```python
from build123d import *

# Parameters (mm, degrees)
BOSS_EXTRUDE1_DEPTH = 1.5
BOSS_EXTRUDE2_START = -10
BOSS_EXTRUDE2_DEPTH = 5
BOSS_EXTRUDE3_START = -50
BOSS_EXTRUDE3_DEPTH = 5
FILLET1_R           = 5
SKETCH4_R           = 1.1
CUT_EXTRUDE1_DEPTH  = 1.5
SKETCH5_R           = 0.85
CUT_EXTRUDE2_DEPTH  = 6


with BuildPart() as part:
    # Sketch1 → Boss-Extrude1 (new body)
    with BuildSketch(Plane(origin=(0, 0, 0), x_dir=(1, 0, 0), z_dir=(0, 1, 0))):
        with BuildLine():
            Line((2.414213562, 0), (69.385786438, 0))
            ThreePointArc((69.385786438, 0), (69.794034728, 0.211324865), (69.857190958, 0.666666667))
            ThreePointArc((69.857190958, 0.666666667), (70.092893219, 1.707106781), (71.133333333, 1.942809042))
            ThreePointArc((71.133333333, 1.942809042), (71.588675135, 2.005965272), (71.8, 2.414213562))
            Line((71.8, 2.414213562), (71.8, 34.385786438))
            ThreePointArc((71.8, 34.385786438), (71.588675135, 34.794034728), (71.133333333, 34.857190958))
            ThreePointArc((71.133333333, 34.857190958), (70.092893219, 35.092893219), (69.857190958, 36.133333333))
            ThreePointArc((69.857190958, 36.133333333), (69.794034728, 36.588675135), (69.385786438, 36.8))
            Line((69.385786438, 36.8), (2.414213562, 36.8))
            ThreePointArc((2.414213562, 36.8), (2.005965272, 36.588675135), (1.942809042, 36.133333333))
            ThreePointArc((1.942809042, 36.133333333), (1.707106781, 35.092893219), (0.666666667, 34.857190958))
            ThreePointArc((0.666666667, 34.857190958), (0.211324865, 34.794034728), (0, 34.385786438))
            Line((0, 34.385786438), (0, 2.414213562))
            ThreePointArc((0, 2.414213562), (0.211324865, 2.005965272), (0.666666667, 1.942809042))
            ThreePointArc((0.666666667, 1.942809042), (1.707106781, 1.707106781), (1.942809042, 0.666666667))
            ThreePointArc((1.942809042, 0.666666667), (2.005965272, 0.211324865), (2.414213562, 0))
        make_face()
    extrude(amount=BOSS_EXTRUDE1_DEPTH)

    # Sketch3 → Boss-Extrude2 (add)
    with BuildSketch(Plane.ZY.offset(BOSS_EXTRUDE2_START)):
        with BuildLine():
            Line((-12.854731747, 0), (-18.4, 0))
            ThreePointArc((-18.4, 0), (-13.582214371, -17.687731165), (-26.704575482, -4.886538603))
            Line((-26.704575482, -4.886538603), (-31.425470843, -1.179783346))
            Line((-31.425470843, -1.179783346), (-32.35181379, -2.359566693))
            Line((-32.35181379, -2.359566693), (-28.576454789, -5.323905182))
            ThreePointArc((-28.576454789, -5.323905182), (-14.871832802, -19.918830847), (-12.854731747, 0))
        make_face()
        with BuildLine():
            Line((-18.4, 0), (-30.499127896, 0))
            Line((-30.499127896, 0), (-25.871961194, -3.633161336))
            ThreePointArc((-25.871961194, -3.633161336), (-22.554216695, -0.956436127), (-18.4, 0))
        make_face()
    extrude(amount=-BOSS_EXTRUDE2_DEPTH)

    # Sketch3_3 → Boss-Extrude3 (add)
    with BuildSketch(Plane.ZY.offset(BOSS_EXTRUDE3_START)):
        with BuildLine():
            Line((-18.4, 0), (-30.499127896, 0))
            Line((-30.499127896, 0), (-25.871961194, -3.633161336))
            ThreePointArc((-25.871961194, -3.633161336), (-22.554216695, -0.956436127), (-18.4, 0))
        make_face()
        with BuildLine():
            Line((-12.854731747, 0), (-18.4, 0))
            ThreePointArc((-18.4, 0), (-13.582214371, -17.687731165), (-26.704575482, -4.886538603))
            Line((-26.704575482, -4.886538603), (-31.425470843, -1.179783346))
            Line((-31.425470843, -1.179783346), (-32.35181379, -2.359566693))
            Line((-32.35181379, -2.359566693), (-28.576454789, -5.323905182))
            ThreePointArc((-28.576454789, -5.323905182), (-14.871832802, -19.918830847), (-12.854731747, 0))
        make_face()
    extrude(amount=-BOSS_EXTRUDE3_DEPTH)

    # Fillet1
    fillet1_edges = [part.edges().sort_by_distance(p)[0] for p in [
        (12.5, 0, -12.854731747),
        (52.5, 0, -12.854731747),
    ]]
    fillet(fillet1_edges, radius=FILLET1_R)

    # Sketch4 → Cut-Extrude1 (cut)
    with BuildSketch(Plane(origin=(0, -17.173792622, -13.484528084), x_dir=(1, 0, 0), z_dir=(0, -0.7865222309713126, -0.6175619646544867))):
        with Locations(Location((12.5, -21.609183849, 0), (0, 0, 270))):
            Circle(SKETCH4_R)
        with Locations(Location((52.5, -21.609183849, 0), (0, 0, 270))):
            Circle(SKETCH4_R)
    extrude(amount=-CUT_EXTRUDE1_DEPTH, mode=Mode.SUBTRACT)

    # Sketch5 → Cut-Extrude2 (cut)
    with BuildSketch(Plane(origin=(0, -17.173792622, -13.484528084), x_dir=(1, 0, 0), z_dir=(0, -0.7865222309713126, -0.6175619646544867))):
        with Locations(Location((12.5, -21.609183849, 0), (0, 0, 270))):
            Circle(SKETCH5_R)
        with Locations(Location((52.5, -21.609183849, 0), (0, 0, 270))):
            Circle(SKETCH5_R)
    extrude(amount=-CUT_EXTRUDE2_DEPTH, mode=Mode.SUBTRACT)


solid = part.part
```
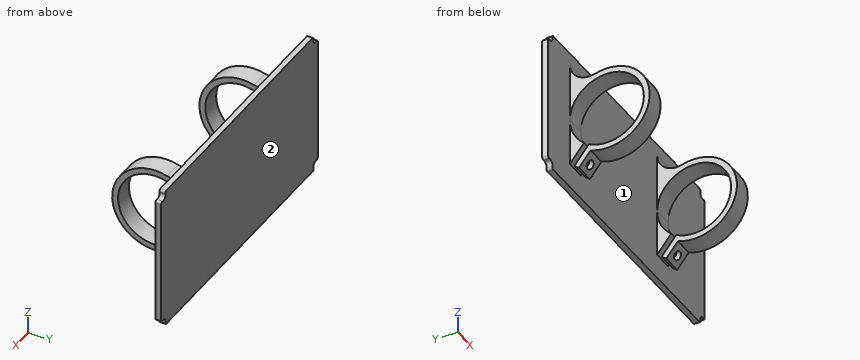
Part model, mm, in its own coordinate system. Face numbers are marked on the shaded views. Give positions to 0.01 mm unless a question says otherwise; leave off trailing zeros. Order: outer loops, then holes, each group sorted by start corner. A loop starts at its lowest first (then second) coordinate and runs counter-clockwise, first axis right, second up. Notation, with made-up numbers: M 27.25,48.25 L 65.25,48.25 A22 ccw 65.25,82.25 Z; hole C 64,73.5 d6. An arc over 180 degrees is marked long. Use a Markdown table: item, result. Add a question column.
(1) Probe line 1 along Y through (x, z) = (53.8, -18.4); line 2 along Z through (x, y) = (51.2, -9.5); line 3 along X through (y, z) = (-13.75, -9). List the from-to ranges inside material, lowest first. Write a range as [from, to].
(2) Saw through at B-B, the plane z = -20.5. Give the cut face in (x, y), and give its area (3 significant figures).
(3) Mould opens along X. For the marked faces 1 and 2 say: +X half, -X half, draft (parallel to the pull), parting line (faces both ways), or undercut.
(4) Saw through at D-D, the plane z = -13. Give the cut face in (x, y), and give its area (3 significant figures).
(5) Saw through at C-C, the plane y = -16.75. Give the cut face in (x, z), and give its area (3 significant figures).
(6) Drop flat-ended pins along their axis: P1, Ø1.1, axis at y = -1, z = -24, coming from the +X side; P2, Ø10, axis at y = -6, z = -15.5, coming from the -X side; P3, Ø5, axis at x = 13.5, z = -32, coming from the -Y side. Give the stop position or say it passes through.
(7) Saw through at A-A, the plane y = -9.5. Give the cut face in (x, z).
Answer key:
| question | item | result |
|---|---|---|
| 1 | line 1 | [-20.5, -19], [0, 1.5] |
| 1 | line 2 | [-29.4, -27.9], [-8.9, -7.4] |
| 1 | line 3 | [10, 15], [50, 55] |
| 2 | outline | M 0,0 L 10,0 L 10,-0.24 L 15,-0.24 L 15,0 L 50,0 L 50,-0.24 L 55,-0.24 L 55,0 L 71.8,0 L 71.8,1.5 L 0,1.5 Z; M 10,-20.3 L 15,-20.3 L 15,-18.76 L 10,-18.76 Z; M 50,-20.3 L 55,-20.3 L 55,-18.76 L 50,-18.76 Z |
| 2 | area | 125 mm^2 |
| 3 | face 1 | undercut |
| 3 | face 2 | draft |
| 4 | outline | M 0,0 L 10,0 L 10,-1.68 L 15,-1.68 L 15,0 L 50,0 L 50,-1.68 L 55,-1.68 L 55,0 L 71.8,0 L 71.8,1.5 L 0,1.5 Z; M 10,-19.08 L 15,-19.08 L 15,-17.32 L 10,-17.32 Z; M 50,-19.08 L 55,-19.08 L 55,-17.32 L 50,-17.32 Z |
| 4 | area | 142 mm^2 |
| 5 | outline | M 10,-26.67 L 15,-26.67 L 15,-24.54 L 10,-24.54 Z; M 10,-12.26 L 15,-12.26 L 15,-10.13 L 10,-10.13 Z; M 50,-26.67 L 55,-26.67 L 55,-24.54 L 50,-24.54 Z; M 50,-12.26 L 55,-12.26 L 55,-10.13 L 50,-10.13 Z |
| 5 | area | 42.7 mm^2 |
| 6 | P1 | x = 55 |
| 6 | P2 | x = 10 |
| 6 | P3 | y = -4.6 |
| 7 | outline | M 10,-29.4 L 15,-29.4 L 15,-27.9 L 10,-27.9 Z; M 10,-8.9 L 15,-8.9 L 15,-7.4 L 10,-7.4 Z; M 50,-29.4 L 55,-29.4 L 55,-27.9 L 50,-27.9 Z; M 50,-8.9 L 55,-8.9 L 55,-7.4 L 50,-7.4 Z |
